Read the model definition and answer for the solid it produces. Units are mm, in the model's axes. Face numbers are marked on the shaded views. Coordinates: 2 decimals unless noted, no trailing zeros. Write each loop counter-clockwise with the first axis right and the second up, starting at its lowest first coordinate (ties: lowest second). Pieces come first, ordered by that corner, then holes.
(1) The part is cut by section D-D, the plane x = 25.5. Determine the outline of the cut face in (y, z).
(2) The part is cut by section C-C, the plane y = 74.5. Determine the outline of the cut face in (x, z), and give its area (3 significant figures).
(3) Determine the mould class of the marked faces 1, 2, 3 and 4 for opening direction X: pulls with the +X half, pulls with the -X half, needs draft (parallel to the pull), parting line crosses it, or undercut.
(4) The part is cut by section B-B, the plane x = 59. Determine the outline of the cut face in (y, z).
(5) Given pin 1 (2.5 mm diameter, centred on x = 15.25, y = 53.98, fed in from +Z); pin 2 (12 mm diameter, centred on x = 48.25, y = 34.92, fed in from +Z); pin 3 (2 mm diameter, centred on x = 31.5, y = 27, fed in from +Z), each flat-ended and moving along its own axis, determine where each tip first touches the part or whether it passes through.
(6) The part is cut by section A-A, the plane y = 25.4. Determine the outline of the cut face in (x, z), and give its area (3 significant figures).
(7) Straight lines are drawn through the part: line 1 along Y through (x, z) = (31.75, 5.85); line 2 along Y through (x, z) = (48, 4); line 3 along X through (y, z) = (82.5, 8). For each, find the intervals that lie inside material, in ascending order.
```python
from build123d import *

# Parameters (mm, degrees)
F0_W     = 63.5
F0_H     = 88.9
F1_DEPTH = 7.62
F2_R     = 2.286
F3_DEPTH = 25.4
F4_R     = 3.683
F4_R_2   = 2.286
F5_DEPTH = 5.08
F7_DEPTH = 1


with BuildPart() as f1:
    # F0 (on Top) → F1 (new body)
    with BuildSketch(Plane.XY):
        with Locations((31.75, 44.45)):
            Rectangle(F0_W, F0_H)
    extrude(amount=F1_DEPTH)

    # F2 (on face) → F3 (cut)
    with BuildSketch(Plane.XY.offset(7.62)):
        with BuildLine():
            ThreePointArc((34.036, 63.5), (30.1335538982, 65.1164461018), (31.75, 61.214))
            ThreePointArc((31.75, 61.214), (33.3664461018, 61.8835538982), (34.036, 63.5))
        make_face()
        with Locations((31.75, 25.4)):
            Circle(F2_R)
        with BuildLine():
            Line((48.2477839421, 34.925), (48.2477839421, 37.211))
            ThreePointArc((48.2477839421, 37.211), (46.6313378403, 36.5414461018), (45.9617839421, 34.925))
            Line((45.9617839421, 34.925), (48.2477839421, 34.925))
        make_face()
        with BuildLine():
            ThreePointArc((50.5337839421, 34.925), (49.8642300439, 36.5414461018), (48.2477839421, 37.211))
            Line((48.2477839421, 37.211), (48.2477839421, 34.925))
            Line((48.2477839421, 34.925), (45.9617839421, 34.925))
            ThreePointArc((45.9617839421, 34.925), (48.2477839421, 32.639), (50.5337839421, 34.925))
        make_face()
        with BuildLine():
            Line((48.2477839421, 53.975), (45.9617839421, 53.975))
            ThreePointArc((45.9617839421, 53.975), (46.6313378403, 52.3585538982), (48.2477839421, 51.689))
            Line((48.2477839421, 51.689), (48.2477839421, 53.975))
        make_face()
        with BuildLine():
            ThreePointArc((50.5337839421, 53.975), (48.2477839421, 56.261), (45.9617839421, 53.975))
            Line((45.9617839421, 53.975), (48.2477839421, 53.975))
            Line((48.2477839421, 53.975), (48.2477839421, 51.689))
            ThreePointArc((48.2477839421, 51.689), (49.8642300439, 52.3585538982), (50.5337839421, 53.975))
        make_face()
        with BuildLine():
            Line((15.2522160579, 53.975), (17.5382160579, 53.975))
            ThreePointArc((17.5382160579, 53.975), (13.6357699561, 55.5914461018), (15.2522160579, 51.689))
            Line((15.2522160579, 51.689), (15.2522160579, 53.975))
        make_face()
        with BuildLine():
            ThreePointArc((15.2522160579, 51.689), (16.8686621597, 52.3585538982), (17.5382160579, 53.975))
            Line((17.5382160579, 53.975), (15.2522160579, 53.975))
            Line((15.2522160579, 53.975), (15.2522160579, 51.689))
        make_face()
        with BuildLine():
            ThreePointArc((17.5382160579, 34.925), (16.8686621597, 36.5414461018), (15.2522160579, 37.211))
            Line((15.2522160579, 37.211), (15.2522160579, 34.925))
            Line((15.2522160579, 34.925), (17.5382160579, 34.925))
        make_face()
        with BuildLine():
            Line((15.2522160579, 34.925), (15.2522160579, 37.211))
            ThreePointArc((15.2522160579, 37.211), (13.6357699561, 33.3085538982), (17.5382160579, 34.925))
            Line((17.5382160579, 34.925), (15.2522160579, 34.925))
        make_face()
        with BuildLine():
            ThreePointArc((31.75, 46.736), (30.1335538982, 42.8335538982), (34.036, 44.45))
            ThreePointArc((34.036, 44.45), (33.3664461018, 46.0664461018), (31.75, 46.736))
        make_face()
    extrude(amount=-F3_DEPTH, mode=Mode.SUBTRACT)

    # F4 (on face) → F5 (cut)
    with BuildSketch(Plane.XY.offset(7.62)):
        with Locations((15.2522160579, 34.925)):
            Circle(F4_R)
        with Locations((15.2522160579, 34.925)):
            Circle(F4_R_2, mode=Mode.SUBTRACT)
        with Locations((15.2522160579, 53.975)):
            Circle(F4_R)
        with Locations((15.2522160579, 53.975)):
            Circle(F4_R_2, mode=Mode.SUBTRACT)
        with Locations((31.75, 63.5)):
            Circle(F4_R)
        with Locations((31.75, 63.5)):
            Circle(F4_R_2, mode=Mode.SUBTRACT)
        with Locations((48.2477839421, 53.975)):
            Circle(F4_R)
        with Locations((48.2477839421, 53.975)):
            Circle(F4_R_2, mode=Mode.SUBTRACT)
        with Locations((48.2477839421, 34.925)):
            Circle(F4_R)
        with Locations((48.2477839421, 34.925)):
            Circle(F4_R_2, mode=Mode.SUBTRACT)
        with Locations((31.75, 25.4)):
            Circle(F4_R)
        with Locations((31.75, 25.4)):
            Circle(F4_R_2, mode=Mode.SUBTRACT)
        with Locations((31.75, 44.45)):
            Circle(F4_R)
        with Locations((31.75, 44.45)):
            Circle(F4_R_2, mode=Mode.SUBTRACT)
    extrude(amount=-F5_DEPTH, mode=Mode.SUBTRACT)

    # F6 (on face) → F7 (join)
    with BuildSketch(Plane.XY.offset(7.62)):
        Polygon((6.35, 19.05), (0, 19.05), (0, 0), (19.05, 0), (19.05, 6.35), (6.35, 6.35), align=None)
        Polygon((44.45, 6.35), (44.45, 0), (63.5, 0), (63.5, 19.05), (57.15, 19.05), (57.15, 6.35), align=None)
        Polygon((63.5, 88.9), (44.45, 88.9), (44.45, 82.55), (57.15, 82.55), (57.15, 69.85), (63.5, 69.85), align=None)
        Polygon((0, 88.9), (0, 69.85), (6.35, 69.85), (6.35, 82.55), (19.05, 82.55), (19.05, 88.9), align=None)
    extrude(amount=F7_DEPTH)


solid = f1.part
```
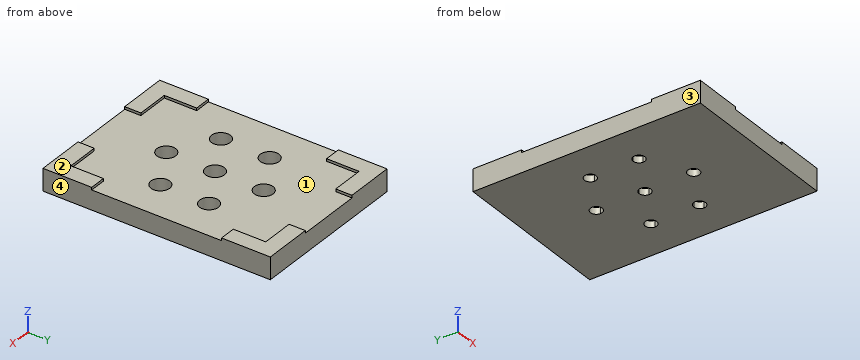
Computed:
1. outline: (0, 0) - (88.9, 0) - (88.9, 7.62) - (0, 7.62) - close
2. outline: (0, 0) - (63.5, 0) - (63.5, 8.62) - (57.15, 8.62) - (57.15, 7.62) - (6.35, 7.62) - (6.35, 8.62) - (0, 8.62) - close
2. area: 497 mm2
3. face 1: undercut
3. face 2: needs draft
3. face 3: pulls with the -X half
3. face 4: pulls with the +X half
4. outline: (0, 0) - (88.9, 0) - (88.9, 8.62) - (69.85, 8.62) - (69.85, 7.62) - (19.05, 7.62) - (19.05, 8.62) - (0, 8.62) - close
5. pin 1: passes through
5. pin 2: stops at z = 7.62
5. pin 3: stops at z = 2.54
6. outline: (0, 0) - (29.46, 0) - (29.46, 2.54) - (28.07, 2.54) - (28.07, 7.62) - (0, 7.62) - close; (34.04, 0) - (63.5, 0) - (63.5, 7.62) - (35.43, 7.62) - (35.43, 2.54) - (34.04, 2.54) - close
6. area: 435 mm2
7. line 1: y = 0 to 21.72, 29.08 to 40.77, 48.13 to 59.82, 67.18 to 88.9
7. line 2: y = 0 to 31.25, 38.6 to 50.3, 57.65 to 88.9
7. line 3: x = 0 to 6.35, 57.15 to 63.5
